from build123d import *

# Parameters (mm, degrees)
SKETCH1_R               = 13
SKETCH1_R_2             = 10
BOSS_EXTRUDE1_DEPTH     = 137.5
SKETCH3_R               = 2.5
CUT_EXTRUDE1_DEPTH      = 14
SKETCH4_R               = 2.65
CUT_EXTRUDE2_DEPTH      = 150
CUT_EXTRUDE2_DEPTH_BACK = 14.0000001


with BuildPart() as part:
    # Sketch1 → Boss-Extrude1 (new body)
    with BuildSketch(Plane.XY):
        Circle(SKETCH1_R)
        Circle(SKETCH1_R_2, mode=Mode.SUBTRACT)
    extrude(amount=BOSS_EXTRUDE1_DEPTH)

    # Sketch3 → Cut-Extrude1 (cut, through all)
    with BuildSketch(Plane(origin=(0, 0, 0), x_dir=(1, 0, 0), z_dir=(0, 1, 0))):
        with Locations((0, -10)):
            Circle(SKETCH3_R)
        with Locations((0, -20)):
            Circle(SKETCH3_R)
    extrude(amount=-CUT_EXTRUDE1_DEPTH, mode=Mode.SUBTRACT)

    # Sketch4 → Cut-Extrude2 (cut, two sides)
    with BuildSketch(Plane(origin=(0, 0, 0), x_dir=(0, 0, -1), z_dir=(0, 1, 0))) as cut_extrude2_sk:
        with Locations((-127.5, 0)):
            Circle(SKETCH4_R)
    extrude(amount=CUT_EXTRUDE2_DEPTH, mode=Mode.SUBTRACT)
    extrude(cut_extrude2_sk.sketch, amount=-CUT_EXTRUDE2_DEPTH_BACK, mode=Mode.SUBTRACT)


solid = part.part
Source: CAD feature listing. Evaluate the final solid. Frame: model axes, mm. A direction names the side the tool comes from. Coordinates: 2 decimals unless noted, no trailing zeros. Loops run counter-clockwise (first coordinate to the right, second up) from the corner with the lowest first, then second, coordinate; pieces in that order, holes last. Notation, with made-up numbers: (18.25, 60.25) -> (23.25, 60.25) arc R13 cw to (23.25, 67.25) -> close; hole circle Ø7 at (87, -25). An arc over 180 degrees is marked (long way). Answer in a Markdown table with one row per item. Add a question column.
Q1. Section A-A on y = 0. Return the cut outline in (x, z), and give its area (3 significant figures).
Q2. Reachability of faces 4 (the face through (-2.234, -11.292, 126.075)), 5 (the face through (-2.5, -11.3, 19.9)) from +Z, -Z, +X, -X, +Y, -Y: full face, straight path, thin tool, end or side. Return the list, or none.
Q3. Section C-C on z = 34.5. Return the cut outline in (x, y), and give its area (3 significant figures).
Q4. Contact query for flat-ended pins moving along their axis: pin 1 Ø10 at (y, z) = (5.5, 74.5) entering from +X; pin 2 Ø6 at (x, z) = (-10.5, 93) entering from -Y; pin 3 Ø4 at (y, z) = (10, 81.5) entering from +X. Output: stop coordinate, or through.
Q5. Pull-direction query (X, two-part tool) for faces 1 (the face through (-2.5, -11.3, 9.9)), 2 (the face through (-2.82, -12.69, 67.79)), 3 (the face through (7, -8, 137.5)); classes: pulls with the +X half, pulls with the -X half, needs draft (parallel to the pull), parting line crosses it, or undercut.
Q6. Section B-B on z = 127.5. Return the cut outline in (x, y).
Q7. Section D-D on z = 20. Return the cut outline in (x, y).
Q8. Ray query, line 1 along Z through (x, y) = (0, -11.75); line 2 along Y through (x, z) = (-0.75, 31); line 3 along Z through (x, y) = (0, 11.45). Return the intervals inside material, ascending.
Computed values:
| question | item | result |
|---|---|---|
| 1 | outline | (-13, 0) -> (-10, 0) -> (-10, 137.5) -> (-13, 137.5) -> close; (10, 0) -> (13, 0) -> (13, 137.5) -> (10, 137.5) -> close |
| 1 | area | 825 mm^2 |
| 2 | face 4 | +Y, -Y |
| 2 | face 5 | -Y |
| 3 | outline | circle Ø26 at (0, 0); hole circle Ø20 at (0, 0) |
| 3 | area | 217 mm^2 |
| 4 | pin 1 | stops at x = 12.99 |
| 4 | pin 2 | stops at y = -10.62 |
| 4 | pin 3 | stops at x = 10.25 |
| 5 | face 1 | undercut |
| 5 | face 2 | parting line crosses it |
| 5 | face 3 | needs draft |
| 6 | outline | (-2.65, -12.73) -> (-2.65, -9.64) arc R10 cw to (-2.65, 9.64) -> (-2.65, 12.73) arc R13 ccw to start; (2.65, -12.73) arc R13 ccw to (2.65, 12.73) -> (2.65, 9.64) arc R10 cw to (2.65, -9.64) -> close |
| 7 | outline | (-2.5, -12.76) -> (-2.5, -9.68) arc R10 cw (long way) to (2.5, -9.68) -> (2.5, -12.76) arc R13 ccw (long way) to start |
| 8 | line 1 | z = 0 to 7.5, 12.5 to 17.5, 22.5 to 124.85, 130.15 to 137.5 |
| 8 | line 2 | y = -12.98 to -9.97, 9.97 to 12.98 |
| 8 | line 3 | z = 0 to 124.85, 130.15 to 137.5 |
